Could you check a few things on this drawing? It's one solid part, dimensions in mm from its lowest x, y, z. A direction names the side the tool comes from. Round coordinates to 2 decimals unless told otherwise and drop trailing zeros. Write each loop counter-clockwise with the first axis right and the second up, starting at its lowest first coordinate (ties: lowest second). Pieces come first, ordered by that corner, then holes. Notation, with made-up numbers: (83, 45.25) -> (87, 45.25) arc R20 cw to (87, 75.25) -> close; hole circle Ø7 at (2, -22). An arc over 180 degrees is marked (long way). Answer in a Markdown table with one row per item.
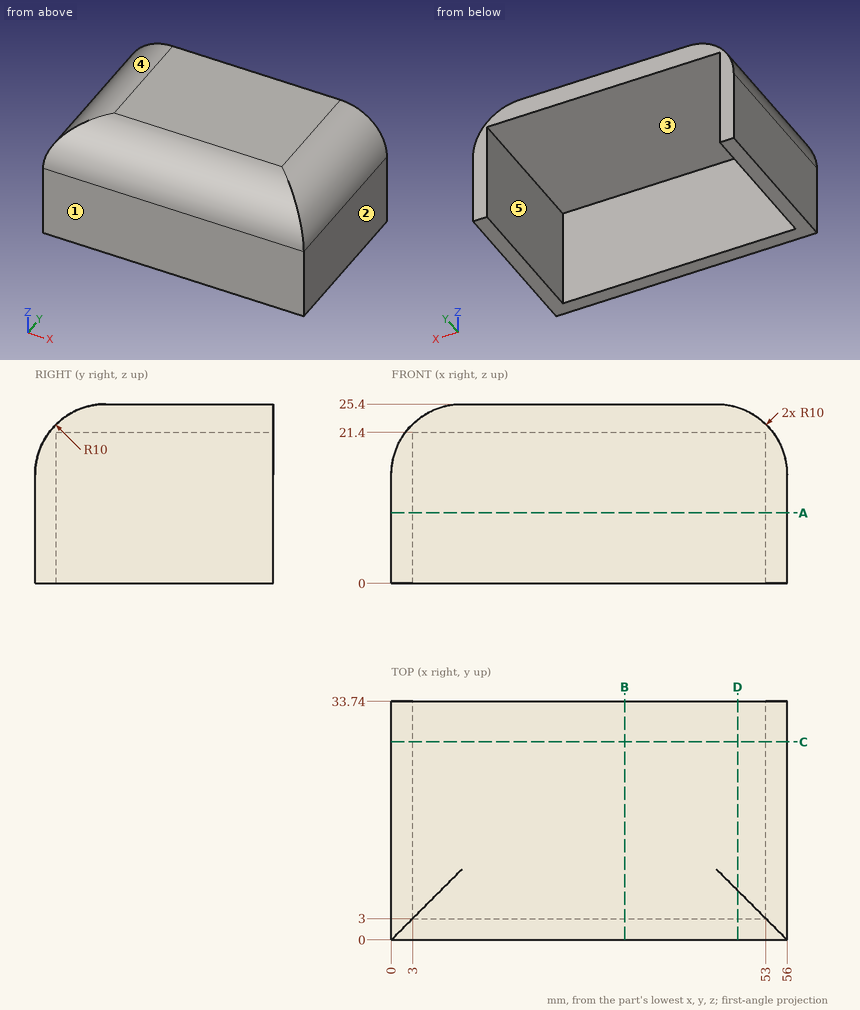
1) For the marked faces 4 and 5, which set-ups out of +Z, -Z, +X, -X, +Y, -Y let a thin tool reach every point of the face, with its end or its side?
Findings:
| item | result |
|---|---|
| face 4 | +Z, -X, +Y, -Y |
| face 5 | -Z, +Y |
2) Imagine slicing it at B-B, the plane x = 33. Please give me the cut outline in (y, z).
Findings:
| item | result |
|---|---|
| outline | (0, 0) -> (3, 0) -> (3, 21.4) -> (33.74, 21.4) -> (33.74, 25.4) -> (10, 25.4) arc R10 ccw to (0, 15.4) -> close |
3) Please list where these lines run through material, in increasing order: line 1 (X direction, y = 27.5, z = 13.25); line 2 (Z direction, x = 26, y = 32.5); line 3 (Y direction, x = 9.5, z = 13.75).
Findings:
| item | result |
|---|---|
| line 1 | x = 0 to 3, 53 to 56 |
| line 2 | z = 21.4 to 25.4 |
| line 3 | y = 0 to 3 |
4) Thinking about a two-plate mould opening in X: for the marked faces 1, 2 and 3, which applies, +X half, -X half, draft (parallel to the pull), parting line (faces both ways), or undercut?
Findings:
| item | result |
|---|---|
| face 1 | draft |
| face 2 | +X half |
| face 3 | undercut |
5) Imagine slicing it at C-C, the plane y = 28. Please give me the cut outline in (x, z).
Findings:
| item | result |
|---|---|
| outline | (0, 0) -> (3, 0) -> (3, 21.4) -> (53, 21.4) -> (53, 0) -> (56, 0) -> (56, 15.4) arc R10 ccw to (46, 25.4) -> (10, 25.4) arc R10 ccw to (0, 15.4) -> close |
6) Imagine slicing it at A-A, the plane z = 10. Please give me the cut outline in (x, y).
Findings:
| item | result |
|---|---|
| outline | (0, 0) -> (56, 0) -> (56, 33.74) -> (53, 33.74) -> (53, 3) -> (3, 3) -> (3, 33.74) -> (0, 33.74) -> close |
7) Imagine slicing it at D-D, the plane x = 49. Please give me the cut outline in (y, z).
Findings:
| item | result |
|---|---|
| outline | (0, 0) -> (3, 0) -> (3, 21.4) -> (33.74, 21.4) -> (33.74, 24.94) -> (7, 24.94) arc R10 ccw to (0, 15.4) -> close |
8) For pin 1 (5 mm diameter, centred on x = 12, z = 15, fed in from +Y); pin 2 (1 mm diameter, centred on x = 19, y = 14.5, fed in from -Z); pin 3 (1.5 mm diameter, centred on y = 14.5, z = 21.5, fed in from -X), each with a flat end and sliding along its axis, tell me the tip position at first contact or that it passes through.
Findings:
| item | result |
|---|---|
| pin 1 | stops at y = 3 |
| pin 2 | stops at z = 21.4 |
| pin 3 | stops at x = 1.55 |
